from build123d import *

# Parameters (mm, degrees)
ESQUISSE1_W             = 40
ESQUISSE1_H             = 55
BOSS_EXTRU_1_DEPTH      = 15
ESQUISSE2_R             = 2
ENL_V_MAT_EXTRU_1_DEPTH = 5
ESQUISSE3_R             = 2
ENL_V_MAT_EXTRU_2_DEPTH = 5


with BuildPart() as part:
    # Esquisse1 → Boss.-Extru.1 (new body)
    with BuildSketch(Plane.XY):
        Rectangle(ESQUISSE1_W, ESQUISSE1_H)
    extrude(amount=BOSS_EXTRU_1_DEPTH)

    # Esquisse2 → Enlèv. mat.-Extru.1 (cut)
    with BuildSketch(Plane(origin=(20, 0, 0), x_dir=(0, 0, -1), z_dir=(1, 0, 0))):
        with Locations((-7.5, 21)):
            Circle(ESQUISSE2_R)
        with Locations((-7.5, -21)):
            Circle(ESQUISSE2_R)
    extrude(amount=-ENL_V_MAT_EXTRU_1_DEPTH, mode=Mode.SUBTRACT)

    # Esquisse3 → Enlèv. mat.-Extru.2 (cut)
    with BuildSketch(Plane.ZY.offset(20)):
        with Locations((7.5, 21)):
            Circle(ESQUISSE3_R)
        with Locations((7.5, -21)):
            Circle(ESQUISSE3_R)
    extrude(amount=-ENL_V_MAT_EXTRU_2_DEPTH, mode=Mode.SUBTRACT)


solid = part.part
Could you check a few things on this model? Use its own coordinates, in mm. A direction names the side the tool comes from. Give positions to 0.01 mm unless a question says otherwise; leave off trailing zeros. Order: outer loops, then holes, each group sorted by start corner. A loop starts at its lowest first (then second) coordinate and runs counter-clockwise, first axis right, second up.
1. For faces 1 (the flat face through (15, -21, 8)), 2 (the cylindrical face through (-17.535, 22.352, 6.026)), 3 (the flat face through (0, -27.5, 7)), which set-ups out of +Z, -Z, +X, -X, +Y, -Y let a thin tool reach every point of the face, with its end or its side?
2. We'd pull the mould along Z, two halves only. Please class faces 4 (the flat face through (0, 0, 15)), 5 (the flat face through (-15, 21, 7)), 6 (the flat face through (-20, 0, 7)), 7 (the flat face through (0, 0, 0)): pulls with the +Z half, pulls with the -Z half, needs draft (parallel to the pull), parting line crosses it, or undercut.
3. Will these pins go through, and if not, where does the flat tip stop? P1, Ø2, axis at y = 21, z = 7.5, coming from the +X side; P2, Ø3.5, axis at y = 21, z = 7.5, coming from the -X side.
4. Suppose I cut it at A-A (z = 7.5). List the corners of the cut face in (x, y) for me.
5. I need wall thicknesses on L1, parallel to Y at x = 18.15, z = 7.5; L2, parallel to X at y = -19.5, z = 7.25; L3, parallel to Z at x = -15.5, y = 22.5. Which ranges of each line are inside material? Lowest first, please.
6. Suppose I cut it at B-B (y = -21). List the corners of the cut face in (x, z) for me.
Solved:
1. face 1: +X
1. face 2: -X
1. face 3: +Z, -Z, +X, -X, -Y
2. face 4: pulls with the +Z half
2. face 5: undercut
2. face 6: needs draft
2. face 7: pulls with the -Z half
3. P1: stops at x = 15
3. P2: stops at x = -15
4. outline: (-20, -27.5) - (20, -27.5) - (20, -23) - (15, -23) - (15, -19) - (20, -19) - (20, 19) - (15, 19) - (15, 23) - (20, 23) - (20, 27.5) - (-20, 27.5) - (-20, 23) - (-15, 23) - (-15, 19) - (-20, 19) - (-20, -19) - (-15, -19) - (-15, -23) - (-20, -23) - close
5. L1: y = -27.5 to -23, -19 to 19, 23 to 27.5
5. L2: x = -15 to 15
5. L3: z = 0 to 6.18, 8.82 to 15
6. outline: (-20, 0) - (20, 0) - (20, 5.5) - (15, 5.5) - (15, 9.5) - (20, 9.5) - (20, 15) - (-20, 15) - (-20, 9.5) - (-15, 9.5) - (-15, 5.5) - (-20, 5.5) - close
